Check sheet for the modelled part. Datum: model origin and axes. Units: mm. Coordinates: 2 decimals unless noted, no trailing zeros. Write each loop counter-clockwise with the first axis right and the second up, starting at its lowest first coordinate (ties: lowest second). Pieces come first, ordered by that corner, then holes. Notation, with made-up numbers: M 51,-8 L 80,-8 A16 cw 80,5 Z; hole C 85,69.25 d11. An arc over 180 degrees is marked long. Answer as CSV lines item,"result". Start each with the question number.
Q1. Thickness scan on line 1 along Y through (x, z) = (0.75, 0); line 2 along Z through (x, y) = (0.25, 40.25); line 3 along X through (y, z) = (71, 3.25). Record the ranges inside material, lowest first. Write a range as from..to.
Q2. Sectioned sample at B-B, the plane x = 0. Record the cut outline in (y, z) (3 decimals).
Q3. Sectioned sample at C-C, the plane y = 40.25. Record the cut outline in (x, z) (3 decimals).
Q4. Sectioned sample at A-A, the plane z = 0. Record the cut outline in (x, y) (3 decimals).
Q5. Sectioned sample at D-D, the plane y = 67. Record the cut outline in (x, z) (3 decimals), then the cut area to 3 significant figures.
Q6. Depth check by flat-ended pin: pin 1 Ø3 at (x, y) = (-2, 57.5) entering from +Z; pin 2 Ø2 at (y, z) = (24.5, 2.5) entering from +X; pin 3 Ø4 at (x, y) = (-5, 54.5) entering from +Z. Enter the tip coordinate at first touch or a pass-through.
from build123d import *

# Parameters (mm, degrees)
SKETCH1_R               = 7.495
BOSS_EXTRUDE1_DEPTH     = 80.5
CUT_EXTRUDE1_DEPTH      = 82.194827729
CUT_EXTRUDE1_DEPTH_BACK = 82.194827729
SKETCH2_R               = 2.5
CHAMFER1_SIZE           = 0.75


with BuildPart() as part:
    # Sketch1 → Boss-Extrude1 (new body)
    with BuildSketch(Plane(origin=(0, 0, 0), x_dir=(1, 0, 0), z_dir=(0, 1, 0))):
        with Locations(Location((0, 0, 0), (0, 0, 270))):
            Circle(SKETCH1_R)
    extrude(amount=BOSS_EXTRUDE1_DEPTH)

    # Sketch2 → Cut-Extrude1 (cut, two sides: drawn at the far end of the back side and taken through both)
    with BuildSketch(Plane(origin=(0, 0, 0), x_dir=(0, 0, -1), z_dir=(1, 0, 0)).offset(-CUT_EXTRUDE1_DEPTH_BACK)):
        with Locations((0, 40.25)):
            Circle(SKETCH2_R)
    extrude(amount=CUT_EXTRUDE1_DEPTH + CUT_EXTRUDE1_DEPTH_BACK, mode=Mode.SUBTRACT)

    # Chamfer1
    chamfer1_edges = [part.edges().sort_by_distance(p)[0] for p in [
        (0, 0, -7.495),
        (0, 80.5, -7.495),
    ]]
    chamfer(chamfer1_edges, length=CHAMFER1_SIZE)


solid = part.part
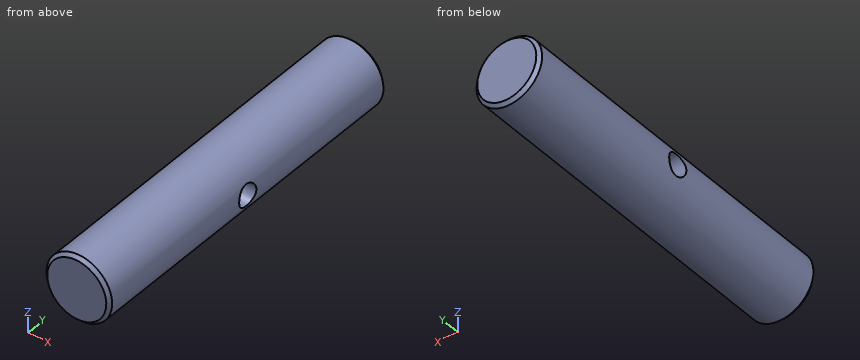
Output:
1,line 1,"y = 0..37.75, 42.75..80.5"
1,line 2,"z = -7.49..-2.5, 2.5..7.49"
1,line 3,"x = -6.75..6.75"
2,outline,"M 0,-6.745 L 0.75,-7.495 L 79.75,-7.495 L 80.5,-6.745 L 80.5,6.745 L 79.75,7.495 L 0.75,7.495 L 0,6.745 Z; hole C 40.25,0 d5"
3,outline,"M -7.066,-2.5 A7.495 ccw 7.066,-2.5 Z; M -7.066,2.5 L 7.066,2.5 A7.495 ccw Z"
4,outline,"M -7.495,0.75 L -6.745,0 L 6.745,0 L 7.495,0.75 L 7.495,37.75 L -7.495,37.75 Z; M -7.495,42.75 L 7.495,42.75 L 7.495,79.75 L 6.745,80.5 L -6.745,80.5 L -7.495,79.75 Z"
5,outline,"C 0,0 d14.99"
5,area,"176 mm^2"
6,pin 1,"stops at z = 7.48"
6,pin 2,"stops at x = 7.34"
6,pin 3,"stops at z = 6.87"
